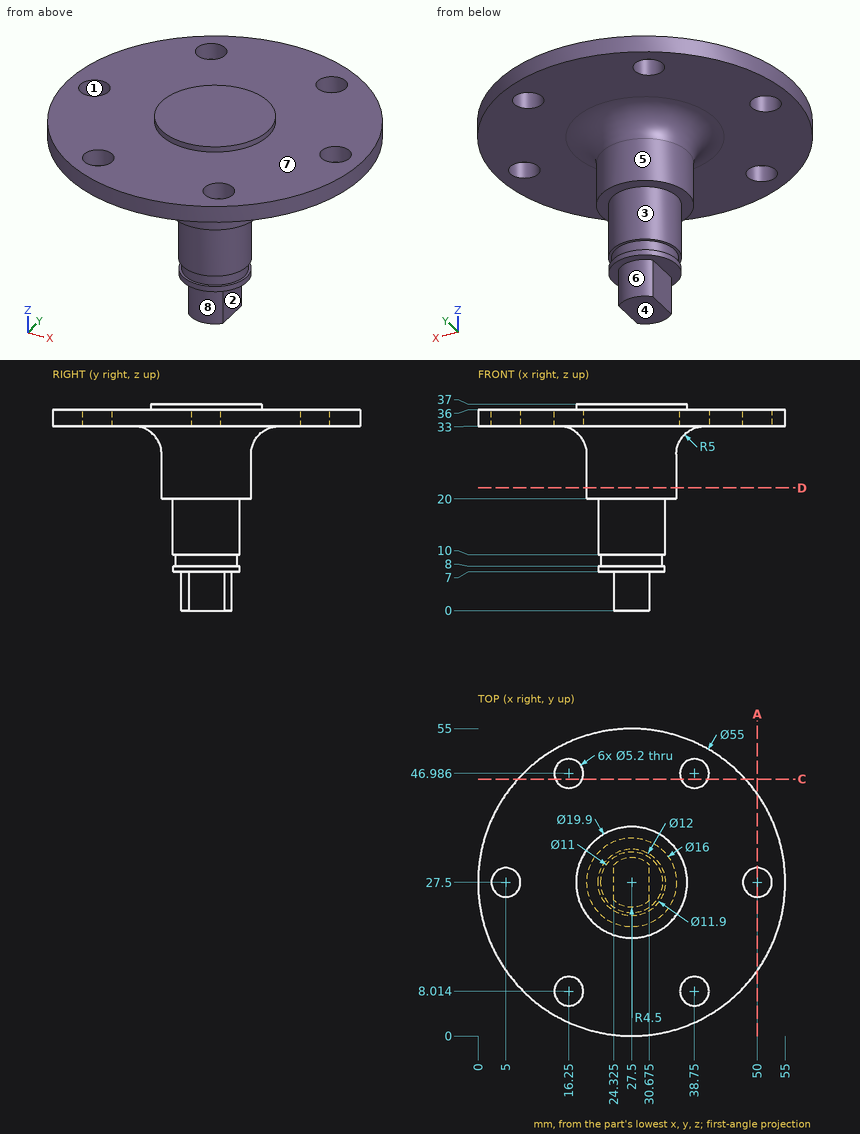
Verification items for this drawing (mm, ordinates from the low corner). A direction names the side the tool comes from. Round coordinates to 2 decimals unless told otherwise and drop trailing zeros. Write each loop counter-clockwise with the first axis right and the second up, starting at its lowest first coordinate (ties: lowest second). Pieces come first, ordered by that corner, then holes. Notation, with made-up numbers: (45, 20) - (98, 20) arc R24 ccw to (98, 43) - close; hole circle Ø3 at (27, -2.75). An arc over 180 degrees is marked (long way). Answer as a JSON object with one key per item and string values. Group by question number.
Q1. Tool access check on the marked faces 5, 6, 7 and 8. Record the directions out of +Z, -Z, +X, -X, +Y, -Y that give a thin tool (end or side, any length) a straight path to the whole face; none if there is none.
Q2. Go/stop test with flat-tipped pins: pin 1 Ø6 at (x, y) = (27.5, 29.5) entering from -Z; pin 2 Ø10 at (y, z) = (33.5, 24.5) entering from +X; pin 3 Ø12 at (x, y) = (37.5, 13.5) entering from +Z; pin 4 Ø8 at (y, z) = (28, 21) entering from +X. Record where each tip stops, or that it passes through.
Q3. Section check A-A, the plane x = 50. Enter the section's corners in (y, z).
Q4. Thickness scan on line 1 (Y direction, x = 16.25, z = 34.6) (1 decimal); line 2 (Y direction, x = 16, z = 34) (1 decimal); line 3 (Z direction, x = 7.5, y = 26.5). Record the ranges inside material, lowest first.
Q5. Section check C-C, the plane y = 46. Enter the section's corners in (x, z).
Q6. Mould release check, pull along X, two halves, no side actions. Record for the marked faces 1, 2, 3 and 4: released by +X, released by -X, zero draft, split by the parting line, or undercut.
Q7. Section check D-D, the plane z = 22. Enter the section's corners in (x, y), plus the area to 3 significant figures.
Found:
{
 "1": {"face 5": "-Z", "face 6": "-Z, +Y", "face 7": "+Z", "face 8": "-Z, -Y"},
 "2": {"pin 1": "stops at z = 0", "pin 2": "stops at x = 35.44", "pin 3": "stops at z = 36", "pin 4": "stops at x = 35.5"},
 "3": {"outline": "(11.69, 33) - (24.9, 33) - (24.9, 36) - (11.69, 36) - close; (30.1, 33) - (43.31, 33) - (43.31, 36) - (30.1, 36) - close"},
 "4": {"line 1": "y = 2.4 to 5.4, 10.6 to 44.4, 49.6 to 52.6", "line 2": "y = 2.5 to 5.4, 10.6 to 44.4, 49.6 to 52.5", "line 3": "z = 33 to 36"},
 "5": {"outline": "(7.15, 33) - (13.84, 33) - (13.84, 36) - (7.15, 36) - close; (18.66, 33) - (36.34, 33) - (36.34, 36) - (18.66, 36) - close; (41.16, 33) - (47.85, 33) - (47.85, 36) - (41.16, 36) - close"},
 "6": {"face 1": "undercut", "face 2": "released by +X", "face 3": "split by the parting line", "face 4": "zero draft"},
 "7": {"outline": "circle Ø16 at (27.5, 27.5)", "area": "201 mm^2"}
}
